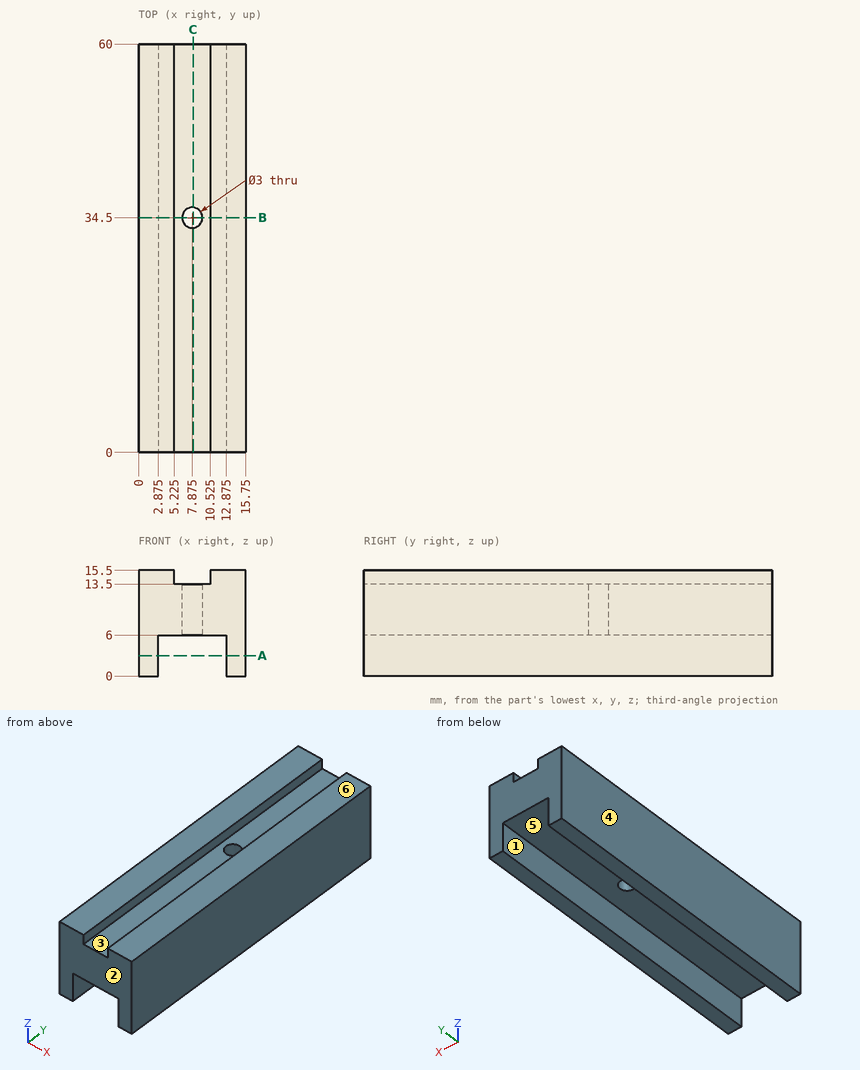
Drawing for the job (mm, zero at the part's lowest x, y, z). A direction names the side the tool comes from. Give positions to 0.01 mm unless a question says otherwise; leave off trailing zeros. Loops run counter-clockwise (first coordinate to the right, second up) from the corner with the lowest first, then second, coordinate; pieces in that order, holes last.
1) Two-plate mould, pull along X, no slides. Class the marked faces 3, 4, 5 and 6: released by +X, released by -X, zero draft, split by the parting line, or undercut.
Values follow:
face 3: undercut
face 4: released by -X
face 5: undercut
face 6: zero draft
2) Band-saw the part on C-C on x = 8. List the corners of the cut face in (y, z).
Values follow:
outline: (0, 6) - (33.01, 6) - (33.01, 13.5) - (0, 13.5) - close; (35.99, 6) - (60, 6) - (60, 13.5) - (35.99, 13.5) - close
3) Band-saw the part on B-B on y = 34.5. List the corners of the cut face in (x, z) (3 decimals).
Values follow:
outline: (0, 0) - (2.875, 0) - (2.875, 6) - (6.375, 6) - (6.375, 13.5) - (5.225, 13.5) - (5.225, 15.5) - (0, 15.5) - close; (9.375, 6) - (12.875, 6) - (12.875, 0) - (15.75, 0) - (15.75, 15.5) - (10.525, 15.5) - (10.525, 13.5) - (9.375, 13.5) - close
4) Drop a flat-ended pin along its axis: P1, Ø5, axis at x = 8, y = 18, coming from the -Z side. Give the stop position or say it passes through.
Values follow:
P1: stops at z = 6
5) Band-saw the part on A-A on z = 3. List the corners of the cut face in (x, y) (3 decimals), then the cut area to 3 significant figures.
Values follow:
outline: (0, 0) - (2.875, 0) - (2.875, 60) - (0, 60) - close; (12.875, 0) - (15.75, 0) - (15.75, 60) - (12.875, 60) - close
area: 345 mm2
6) 3-axis set-ups, long thin cutter, end or side, ignore diameter. For the marked faces 1 and 2: which of +Z, -Z, +X, -X, +Y, -Y reach the whole face in a straight line?
Values follow:
face 1: -Z, +Y, -Y
face 2: +Z, -Z, +X, -X, -Y
7) Probe line 1 along X through (y, z) = (12, 1.5) (3 decimals); line 2 along Z through (x, y) = (9.75, 42); line 3 along Z through (x, y) = (11.75, 33). List the from-to ranges inside material, lowest first.
Values follow:
line 1: x = 0 to 2.875, 12.875 to 15.75
line 2: z = 6 to 13.5
line 3: z = 6 to 15.5
